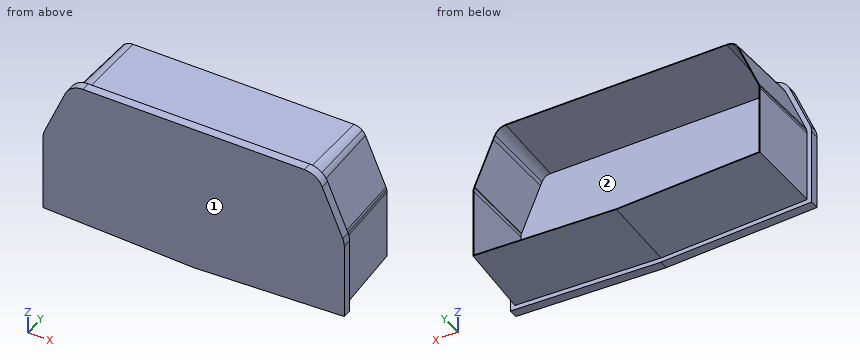
```python
from build123d import *

# Parameters (mm, degrees)
F1_DEPTH = 3
F2_DEPTH = 25
F2_TAPER = 2


with BuildPart() as f1:
    # F0 (on Front) → F1 (new body)
    with BuildSketch(Plane.XZ):
        with BuildLine():
            Line((-50, -13.9400455604), (0, -15.9801289749))
            Line((0, -15.9801289749), (50, -13.9400455604))
            Line((50, -13.9400455604), (50, 11.4815801105))
            ThreePointArc((50, 11.4815801105), (49.8692221387, 12.7788886118), (49.48215097, 14.0239942728))
            Line((49.48215097, 14.0239942728), (42.674322517, 30.0424141622))
            ThreePointArc((42.674322517, 30.0424141622), (40.2785560736, 32.9210558037), (36.692171547, 34))
            Line((36.692171547, 34), (-36.692171547, 34))
            ThreePointArc((-36.692171547, 34), (-40.2785560736, 32.9210558037), (-42.674322517, 30.0424141622))
            Line((-42.674322517, 30.0424141622), (-49.48215097, 14.0239942728))
            ThreePointArc((-49.48215097, 14.0239942728), (-49.8692221387, 12.7788886118), (-50, 11.4815801105))
            Line((-50, 11.4815801105), (-50, -13.9400455604))
        make_face()
        with BuildLine():
            Line((48.5, 11.4815801105), (48.5, -12.5))
            Line((48.5, -12.5), (0, -14.4788809121))
            Line((0, -14.4788809121), (-48.5, -12.5))
            Line((-48.5, -12.5), (-48.5, 11.4815801105))
            ThreePointArc((-48.5, 11.4815801105), (-48.4737268325, 11.9934799011), (-48.3951834418, 12.5))
            ThreePointArc((-48.3951834418, 12.5), (-48.2714890929, 12.9758665077), (-48.1016545923, 13.4372833123))
            Line((-48.1016545923, 13.4372833123), (-41.2938261393, 29.4557032017))
            ThreePointArc((-41.2938261393, 29.4557032017), (-40.7473349126, 30.4250042869), (-40, 31.249436081))
            ThreePointArc((-40, 31.249436081), (-38.4603372059, 32.1769210173), (-36.692171547, 32.5))
            Line((-36.692171547, 32.5), (0, 32.5))
            Line((0, 32.5), (36.692171547, 32.5))
            ThreePointArc((36.692171547, 32.5), (38.4603372059, 32.1769210173), (40, 31.249436081))
            ThreePointArc((40, 31.249436081), (40.7473349126, 30.4250042869), (41.2938261393, 29.4557032017))
            Line((41.2938261393, 29.4557032017), (48.1016545923, 13.4372833123))
            ThreePointArc((48.1016545923, 13.4372833123), (48.2714890929, 12.9758665077), (48.3951834418, 12.5))
            ThreePointArc((48.3951834418, 12.5), (48.4737268325, 11.9934799011), (48.5, 11.4815801105))
        make_face(mode=Mode.SUBTRACT)
        with BuildLine():
            Line((0, 12.5), (0, -12.4772168282))
            Line((0, -12.4772168282), (46.5, -10.5799392527))
            Line((46.5, -10.5799392527), (46.5, 11.4815801105))
            ThreePointArc((46.5, 11.4815801105), (46.4551261591, 11.9985224514), (46.3218470775, 12.5))
            Line((46.3218470775, 12.5), (40, 12.5))
            Line((40, 12.5), (0, 12.5))
        make_face()
        with BuildLine():
            Line((-46.5, -10.5799392527), (0, -12.4772168282))
            Line((0, -12.4772168282), (0, 12.5))
            Line((0, 12.5), (-40, 12.5))
            Line((-40, 12.5), (-46.3218470775, 12.5))
            ThreePointArc((-46.3218470775, 12.5), (-46.4551261591, 11.9985224514), (-46.5, 11.4815801105))
            Line((-46.5, 11.4815801105), (-46.5, -10.5799392527))
        make_face()
        with BuildLine():
            Line((-40, 12.5), (0, 12.5))
            Line((0, 12.5), (0, 30.5))
            Line((0, 30.5), (-36.692171547, 30.5))
            ThreePointArc((-36.692171547, 30.5), (-38.3474259439, 30.0020257556), (-39.4531643024, 28.673421921))
            Line((-39.4531643024, 28.673421921), (-40, 27.3867496913))
            Line((-40, 27.3867496913), (-40, 12.5))
        make_face()
        with BuildLine():
            Line((0, 30.5), (0, 12.5))
            Line((0, 12.5), (40, 12.5))
            Line((40, 12.5), (40, 27.3867496913))
            Line((40, 27.3867496913), (39.4531643024, 28.673421921))
            ThreePointArc((39.4531643024, 28.673421921), (38.3474259439, 30.0020257556), (36.692171547, 30.5))
            Line((36.692171547, 30.5), (0, 30.5))
        make_face()
        with BuildLine():
            Line((0, -12.5), (48.5, -12.5))
            Line((48.5, -12.5), (48.5, 11.4815801105))
            ThreePointArc((48.5, 11.4815801105), (48.4737268325, 11.9934799011), (48.3951834418, 12.5))
            Line((48.3951834418, 12.5), (46.3218470775, 12.5))
            ThreePointArc((46.3218470775, 12.5), (46.4551261591, 11.9985224514), (46.5, 11.4815801105))
            Line((46.5, 11.4815801105), (46.5, -10.5799392527))
            Line((46.5, -10.5799392527), (0, -12.4772168282))
            Line((0, -12.4772168282), (0, -12.5))
        make_face()
        with BuildLine():
            Line((-48.5, -12.5), (0, -12.5))
            Line((0, -12.5), (0, -12.4772168282))
            Line((0, -12.4772168282), (-46.5, -10.5799392527))
            Line((-46.5, -10.5799392527), (-46.5, 11.4815801105))
            ThreePointArc((-46.5, 11.4815801105), (-46.4551261591, 11.9985224514), (-46.3218470775, 12.5))
            Line((-46.3218470775, 12.5), (-48.3951834418, 12.5))
            ThreePointArc((-48.3951834418, 12.5), (-48.4737268325, 11.9934799011), (-48.5, 11.4815801105))
            Line((-48.5, 11.4815801105), (-48.5, -12.5))
        make_face()
        with BuildLine():
            Line((0, 32.5), (0, 30.5))
            Line((0, 30.5), (36.692171547, 30.5))
            ThreePointArc((36.692171547, 30.5), (38.3474259439, 30.0020257556), (39.4531643024, 28.673421921))
            Line((39.4531643024, 28.673421921), (40, 27.3867496913))
            Line((40, 27.3867496913), (40, 31.249436081))
            ThreePointArc((40, 31.249436081), (38.4603372059, 32.1769210173), (36.692171547, 32.5))
            Line((36.692171547, 32.5), (0, 32.5))
        make_face()
        with BuildLine():
            Line((-36.692171547, 30.5), (0, 30.5))
            Line((0, 30.5), (0, 32.5))
            Line((0, 32.5), (-36.692171547, 32.5))
            ThreePointArc((-36.692171547, 32.5), (-38.4603372059, 32.1769210173), (-40, 31.249436081))
            Line((-40, 31.249436081), (-40, 27.3867496913))
            Line((-40, 27.3867496913), (-39.4531643024, 28.673421921))
            ThreePointArc((-39.4531643024, 28.673421921), (-38.3474259439, 30.0020257556), (-36.692171547, 30.5))
        make_face()
        Polygon((0, -14.4788809121), (48.5, -12.5), (0, -12.5), align=None)
        Polygon((0, -14.4788809121), (0, -12.5), (-48.5, -12.5), align=None)
        with BuildLine():
            Line((-46.3218470775, 12.5), (-40, 12.5))
            Line((-40, 12.5), (-40, 27.3867496913))
            Line((-40, 27.3867496913), (-46.2609927554, 12.6550020316))
            ThreePointArc((-46.2609927554, 12.6550020316), (-46.2924955787, 12.5779233244), (-46.3218470775, 12.5))
        make_face()
        with BuildLine():
            Line((40, 12.5), (46.3218470775, 12.5))
            ThreePointArc((46.3218470775, 12.5), (46.2924955787, 12.5779233244), (46.2609927554, 12.6550020316))
            Line((46.2609927554, 12.6550020316), (40, 27.3867496913))
            Line((40, 27.3867496913), (40, 12.5))
        make_face()
        with BuildLine():
            ThreePointArc((-48.1016545923, 13.4372833123), (-48.2714890929, 12.9758665077), (-48.3951834418, 12.5))
            Line((-48.3951834418, 12.5), (-46.3218470775, 12.5))
            ThreePointArc((-46.3218470775, 12.5), (-46.2924955787, 12.5779233244), (-46.2609927554, 12.6550020316))
            Line((-46.2609927554, 12.6550020316), (-40, 27.3867496913))
            Line((-40, 27.3867496913), (-40, 31.249436081))
            ThreePointArc((-40, 31.249436081), (-40.7473349126, 30.4250042869), (-41.2938261393, 29.4557032017))
            Line((-41.2938261393, 29.4557032017), (-48.1016545923, 13.4372833123))
        make_face()
        with BuildLine():
            Line((46.3218470775, 12.5), (48.3951834418, 12.5))
            ThreePointArc((48.3951834418, 12.5), (48.2714890929, 12.9758665077), (48.1016545923, 13.4372833123))
            Line((48.1016545923, 13.4372833123), (41.2938261393, 29.4557032017))
            ThreePointArc((41.2938261393, 29.4557032017), (40.7473349126, 30.4250042869), (40, 31.249436081))
            Line((40, 31.249436081), (40, 27.3867496913))
            Line((40, 27.3867496913), (46.2609927554, 12.6550020316))
            ThreePointArc((46.2609927554, 12.6550020316), (46.2924955787, 12.5779233244), (46.3218470775, 12.5))
        make_face()
    extrude(amount=F1_DEPTH)

    # F0 (on Front) → F2 (join)
    with BuildSketch(Plane.XZ):
        with BuildLine():
            Line((-36.692171547, 30.5), (0, 30.5))
            Line((0, 30.5), (0, 32.5))
            Line((0, 32.5), (-36.692171547, 32.5))
            ThreePointArc((-36.692171547, 32.5), (-38.4603372059, 32.1769210173), (-40, 31.249436081))
            Line((-40, 31.249436081), (-40, 27.3867496913))
            Line((-40, 27.3867496913), (-39.4531643024, 28.673421921))
            ThreePointArc((-39.4531643024, 28.673421921), (-38.3474259439, 30.0020257556), (-36.692171547, 30.5))
        make_face()
        with BuildLine():
            ThreePointArc((-48.1016545923, 13.4372833123), (-48.2714890929, 12.9758665077), (-48.3951834418, 12.5))
            Line((-48.3951834418, 12.5), (-46.3218470775, 12.5))
            ThreePointArc((-46.3218470775, 12.5), (-46.2924955787, 12.5779233244), (-46.2609927554, 12.6550020316))
            Line((-46.2609927554, 12.6550020316), (-40, 27.3867496913))
            Line((-40, 27.3867496913), (-40, 31.249436081))
            ThreePointArc((-40, 31.249436081), (-40.7473349126, 30.4250042869), (-41.2938261393, 29.4557032017))
            Line((-41.2938261393, 29.4557032017), (-48.1016545923, 13.4372833123))
        make_face()
        with BuildLine():
            Line((-48.5, -12.5), (0, -12.5))
            Line((0, -12.5), (0, -12.4772168282))
            Line((0, -12.4772168282), (-46.5, -10.5799392527))
            Line((-46.5, -10.5799392527), (-46.5, 11.4815801105))
            ThreePointArc((-46.5, 11.4815801105), (-46.4551261591, 11.9985224514), (-46.3218470775, 12.5))
            Line((-46.3218470775, 12.5), (-48.3951834418, 12.5))
            ThreePointArc((-48.3951834418, 12.5), (-48.4737268325, 11.9934799011), (-48.5, 11.4815801105))
            Line((-48.5, 11.4815801105), (-48.5, -12.5))
        make_face()
        Polygon((0, -14.4788809121), (0, -12.5), (-48.5, -12.5), align=None)
        Polygon((0, -14.4788809121), (48.5, -12.5), (0, -12.5), align=None)
        with BuildLine():
            Line((0, -12.5), (48.5, -12.5))
            Line((48.5, -12.5), (48.5, 11.4815801105))
            ThreePointArc((48.5, 11.4815801105), (48.4737268325, 11.9934799011), (48.3951834418, 12.5))
            Line((48.3951834418, 12.5), (46.3218470775, 12.5))
            ThreePointArc((46.3218470775, 12.5), (46.4551261591, 11.9985224514), (46.5, 11.4815801105))
            Line((46.5, 11.4815801105), (46.5, -10.5799392527))
            Line((46.5, -10.5799392527), (0, -12.4772168282))
            Line((0, -12.4772168282), (0, -12.5))
        make_face()
        with BuildLine():
            Line((46.3218470775, 12.5), (48.3951834418, 12.5))
            ThreePointArc((48.3951834418, 12.5), (48.2714890929, 12.9758665077), (48.1016545923, 13.4372833123))
            Line((48.1016545923, 13.4372833123), (41.2938261393, 29.4557032017))
            ThreePointArc((41.2938261393, 29.4557032017), (40.7473349126, 30.4250042869), (40, 31.249436081))
            Line((40, 31.249436081), (40, 27.3867496913))
            Line((40, 27.3867496913), (46.2609927554, 12.6550020316))
            ThreePointArc((46.2609927554, 12.6550020316), (46.2924955787, 12.5779233244), (46.3218470775, 12.5))
        make_face()
        with BuildLine():
            Line((0, 32.5), (0, 30.5))
            Line((0, 30.5), (36.692171547, 30.5))
            ThreePointArc((36.692171547, 30.5), (38.3474259439, 30.0020257556), (39.4531643024, 28.673421921))
            Line((39.4531643024, 28.673421921), (40, 27.3867496913))
            Line((40, 27.3867496913), (40, 31.249436081))
            ThreePointArc((40, 31.249436081), (38.4603372059, 32.1769210173), (36.692171547, 32.5))
            Line((36.692171547, 32.5), (0, 32.5))
        make_face()
    extrude(amount=-F2_DEPTH, taper=F2_TAPER)


solid = f1.part
```
For this review, take the finished solid that the model builds, in its own axes (mm). Face numbers are marked on the shaded views. Give positions to 0.01 mm unless a question says otherwise; leave off trailing zeros. Order: outer loops, then holes, each group sorted by start corner. A loop starts at its lowest first (then second) coordinate and runs counter-clockwise, first axis right, second up.
1) Take a section at A-A (y = -1). Give the boundary of the cut face in (x, z), then the cut area to 3 significant figures.
2) Wall thickness on line 1 (Y direction, x = 14, z = 23); line 2 (Z direction, x = -10, y = 21.25); line 3 (X direction, y = 14, z = -3.5): over which ranges is each line inside the solid? List them lowest first.
3) The part is to be moulded in two halves that separate along Z. For the marked faces 1 and 2, say which applies: released by +Z, released by -Z, zero draft, split by the parting line, or undercut.
4) Insertion check: pin 1 (1 mm diameter, centred on y = 21, z = -7, fed in from +X); pin 2 (5 mm diameter, centred on x = -14, y = 17.5, fed in from +Z); pin 3 (12 mm diameter, centred on x = -10, y = 10.5, fed in from +Z). Each pin has a flat end and moves straight along its axis. Give the tip position at first contact, or say it passes through.
Derived:
1. outline: (-50, -13.94) - (0, -15.98) - (50, -13.94) - (50, 11.48) arc R6.5 ccw to (49.48, 14.02) - (42.67, 30.04) arc R6.5 ccw to (36.69, 34) - (-36.69, 34) arc R6.5 ccw to (-42.67, 30.04) - (-49.48, 14.02) arc R6.5 ccw to (-50, 11.48) - close
1. area: 4,700 mm2
2. line 1: y = -3 to 0
2. line 2: z = -13.33 to -12.81, 31.24 to 31.76
2. line 3: x = -48.01 to -46.99, 46.99 to 48.01
3. face 1: zero draft
3. face 2: undercut
4. pin 1: stops at x = 47.78
4. pin 2: stops at z = 31.98
4. pin 3: stops at z = 32.34
